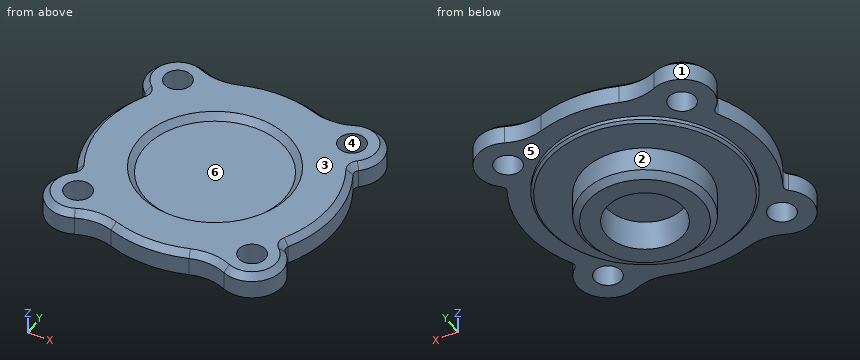
Autodesk Inventor part; units mm, degrees
ref_plane "YZ Plane" through (0, 0, 0) normal (1, 0, 0) x (0, 1, 0)
ref_plane "XZ Plane" through (0, 0, 0) normal (0, 1, 0) x (-1, 0, 0)
ref_plane "XY Plane" through (0, 0, 0) normal (0, 0, 1) x (1, 0, 0)
sketch "Sketch1" plane through (0, 0, 0) normal (0, 0, 1) x (1, 0, 0)
  circle A0 centre (0, 0) radius 10.4775
  circle A1 centre (9.0932, -9.0932) radius 0.9652
  circle A2 centre (-9.0932, 9.0932) radius 0.9652
  circle A3 centre (9.0932, 9.0932) radius 0.9652
  circle A4 centre (-9.0932, -9.0932) radius 0.9652
  arc A5 (11.1694, 6.6911) -> (7.7987, 11.9923) centre (9.0932, 9.0932) ccw
  arc A6 (4.0733, 11.8277) -> (7.7987, 11.9923) centre (5.7275, 16.6309) ccw
  arc A7 (4.0733, 11.8277) -> (-4.0733, 11.8277) centre (0, 0) ccw
  arc A8 (-7.7987, 11.9923) -> (-4.0733, 11.8277) centre (-5.7275, 16.6309) ccw
  arc A9 (-7.7987, 11.9923) -> (-11.1694, 6.6911) centre (-9.0932, 9.0932) ccw
  arc A10 (-11.025, 5.9107) -> (-11.1694, 6.6911) centre (-11.5847, 6.2107) ccw
  arc A11 (-11.025, 5.9107) -> (-11.025, -5.9107) centre (0, 0) ccw
  arc A12 (-11.1694, -6.6911) -> (-11.025, -5.9107) centre (-11.5847, -6.2107) ccw
  arc A13 (-11.1694, -6.6911) -> (-7.7987, -11.9923) centre (-9.0932, -9.0932) ccw
  arc A14 (-4.0733, -11.8277) -> (-7.7987, -11.9923) centre (-5.7275, -16.6309) ccw
  arc A15 (-4.0733, -11.8277) -> (4.0733, -11.8277) centre (0, 0) ccw
  arc A16 (7.7987, -11.9923) -> (4.0733, -11.8277) centre (5.7275, -16.6309) ccw
  arc A17 (7.7987, -11.9923) -> (11.1694, -6.6911) centre (9.0932, -9.0932) ccw
  arc A18 (11.025, -5.9107) -> (11.1694, -6.6911) centre (11.5847, -6.2107) ccw
  arc A19 (11.025, -5.9107) -> (11.025, 5.9107) centre (0, 0) ccw
  arc A20 (11.1694, 6.6911) -> (11.025, 5.9107) centre (11.5847, 6.2107) ccw
  point P0 (0, 0)
extrude "Extrusion1" add sketch "Sketch1" along normal blind 2.54 contours A0 | A1 | A2 | A3 | A4 | A20 A19 A18 A17 A16 A15 A14 A13 A12 A11 A10 A9 A8 A7 A6 A5
sketch "Sketch2" plane through (0, 0, 0) normal (0, 0, -1) x (-1, 0, 0)
  circle A0 centre (0, 0) radius 10.4775
  circle A1 centre (0, 0) radius 10.3505
  dimension "d2" = 0.127
extrude "Extrusion2" add sketch "Sketch2" along normal blind 0.635 contours A1
sketch "Sketch3" plane through (0, 0, -0.635) normal (0, 0, -1) x (-1, 0, 0)
  circle A0 centre (0, 0) radius 4.0005
  circle A1 centre (0, 0) radius 4.0259
  circle A2 centre (0, 0) radius 6.5659
  dimension "d5" = 0.0254
  dimension "d6" = 2.54
extrude "Extrusion3" add sketch "Sketch3" along normal blind 3.175 contours A2
chamfer "Chamfer1" distance 0.635 angle 45 1 edges at (6.5659, 0, -3.81)
chamfer "Chamfer4" distance 0.254 angle 45 1 edges at (10.3505, 0, -0.635)
sketch "Sketch4" plane through (0, 0, 2.54) normal (0, 0, 1) x (1, 0, 0)
  arc A0 (11.1694, 6.6911) -> (7.7987, 11.9923) centre (9.0932, 9.0932) ccw
  arc A1 (-7.7987, 11.9923) -> (-11.1694, 6.6911) centre (-9.0932, 9.0932) ccw
  arc A2 (-11.1694, -6.6911) -> (-7.7987, -11.9923) centre (-9.0932, -9.0932) ccw
  arc A3 (7.7987, -11.9923) -> (11.1694, -6.6911) centre (9.0932, -9.0932) ccw
hole "Hole1" at (9.0932, 9.0932, 2.54) at (-9.0932, 9.0932, 2.54) at (-9.0932, -9.0932, 2.54) at (9.0932, -9.0932, 2.54) direction (0, 0, -1) diameter 2.794 end through all
sketch "Sketch5" plane through (0, 0, 2.54) normal (0, 0, 1) x (1, 0, 0)
  arc A0 (11.025, -5.9107) -> (11.025, 5.9107) centre (0, 0) ccw
  circle A1 centre (0, 0) radius 7.9375
  dimension "d19" = 15.875
extrude "Extrusion4" cut sketch "Sketch5" against normal blind 0.635
chamfer "Chamfer2" distance 0.635 angle 45 1 edges at (-7.9375, 0, 1.905)
chamfer "Chamfer3" distance 0.635 angle 45 16 edges at (12.5095, 0, 2.54) (10.9603, 6.3263, 2.54) (11.7724, 10.7968, 2.54) (5.9517, 11.5558, 2.54) (0, 12.5095, 2.54) (-5.9517, 11.5558, 2.54) (-11.7724, 10.7968, 2.54) (-10.9603, 6.3263, 2.54) (-12.5095, 0, 2.54) (-10.9603, -6.3263, 2.54) (-11.7724, -10.7968, 2.54) (-5.9517, -11.5558, 2.54) (0, -12.5095, 2.54) (5.9517, -11.5558, 2.54) (11.7724, -10.7968, 2.54) (10.9603, -6.3263, 2.54)
properties part number "Crankshaft Cover"
Model file for the job. Use its own axes, mm. Face numbers are marked on the shaded views. A direction names the side the tool comes from. Give positions to 0.01 mm unless a question says otherwise; leave off trailing zeros. Write each loop counter-clockwise with the first axis right and the second up, starting at its lowest first coordinate (ties: lowest second). Pieces come first, ordered by that corner, then holes. Notation, with made-up numbers: (52.5, 65.5) - (59.5, 65.5) arc R32 ccw to (59.5, 98.5) - close; hole circle Ø1 at (50.25, -18.75). An arc over 180 degrees is marked (long way). Answer as CSV lines item,"result".
1. Pin check, flat tips, straight feed: pin 1 (2 mm diameter, centred on x = 9.09, y = 9.09, fed in from -Z); pin 2 (1 mm diameter, centred on x = -8, z = -1, fed in from -Y); pin 3 (3 mm diameter, centred on x = 5, z = -1, fed in from -Y); pin 4 (1 mm diameter, centred on x = -6, z = 0.5, fed in from -Y). Stop position of each tip, or through.
Responses:
pin 1,"passes through"
pin 2,"stops at y = -6.58"
pin 3,"stops at y = -11.89"
pin 4,"stops at y = -11.61"
2. Drill centre lines: L1, parallel to X at y = 9.5, z = 2.25; L2, parallel to Z at x = -3.25, y = -3.5 (3 decimals); L3, parallel to Z at x = -9, y = 0 (3 decimals). Where is each one in solid material? Low to high. Write a range as [from, to].
Responses:
L1,"x = [-11.89, -10.43], [-7.76, 7.76], [10.43, 11.89]"
L2,"z = [-3.81, 1.905]"
L3,"z = [-0.635, 2.54]"
3. 3-axis set-ups, long thin cutter, end or side, ignore diameter. For the marked faces 4, 5 and 6: which of +Z, -Z, +X, -X, +Y, -Y reach the whole face in a straight line?
Responses:
face 4,"+Z, -Z"
face 5,"-Z"
face 6,"+Z"
4. Band-saw the part on C-C (z = 1). Write the cut outline in (x, y) (3 decimals).
Responses:
outline,"(-11.169, -6.691) arc R3.175 ccw to (-7.799, -11.992) arc R5.08 cw to (-4.073, -11.828) arc R12.509 ccw to (4.073, -11.828) arc R5.08 cw to (7.799, -11.992) arc R3.175 ccw to (11.169, -6.691) arc R0.635 cw to (11.025, -5.911) arc R12.509 ccw to (11.025, 5.911) arc R0.635 cw to (11.169, 6.691) arc R3.175 ccw to (7.799, 11.992) arc R5.08 cw to (4.073, 11.828) arc R12.509 ccw to (-4.073, 11.828) arc R5.08 cw to (-7.799, 11.992) arc R3.175 ccw to (-11.169, 6.691) arc R0.635 cw to (-11.025, 5.911) arc R12.509 ccw to (-11.025, -5.911) arc R0.635 cw to start; hole circle Ø2.794 at (-9.093, -9.093); hole circle Ø2.794 at (-9.093, 9.093); hole circle Ø2.794 at (9.093, -9.093); hole circle Ø2.794 at (9.093, 9.093)"
5. Band-saw the part on D-D (z = -1.5). Write the cut outline in (x, y).
Responses:
outline,"circle Ø13.13 at (0, 0); hole circle Ø8.05 at (0, 0)"
6. Two-plate mould, pull along Y, no slides. Class the marked faces 1, 2 and 3: +Y half, -Y half, draft (parallel to the pull), parting line (faces both ways), or undercut.
Responses:
face 1,"undercut"
face 2,"parting line"
face 3,"draft"
